Check sheet for the drawn part. Datum: minimum x, y, z corner. Units: mm. Coordinates: 2 decimals unless noted, no trailing zeros. Write each loop counter-clockwise with the first axis right and the second up, starting at its lowest first coordinate (ties: lowest second). Pieces come first, ordered by that corner, then holes. Notation, with made-up numbers: (85.25, 17) -> (131.25, 17) arc R34 cw to (131.25, 51) -> close; hole circle Ø6 at (25, 87.25). An arc over 180 degrees is marked (long way). Answer in a Markdown table with one row per item. Add a question column.
1. Cross-section at B-B on z = 2.1. Record the cut outline in (x, y), and give its area (3 significant figures).
2. Cross-section at D-D on z = 0.35. Record the cut outline in (x, y), and give its area (3 significant figures).
3. Cross-section at A-A on y = 3.75. Record the cut outline in (x, z).
4. Depth check by flat-ended pin: P1, Ø1, axis at x = 3, z = 1, coming from the -Y side; P2, Ø1, axis at x = 2, z = 1, coming from the +Y side. Enter the tip coordinate at first touch or a pass-through.
5. Cross-section at C-C on z = 1.65. Record the cut outline in (x, y).
6. Scan lines: L1, parallel to Y at x = 3.75, z = 1.15; L2, parallel to Z at x = 2.25, y = 4.5; L3, parallel to X at y = 5.25, z = 0.25. Record each from-to range of solid material in increasing order. Write a range as from..to.
7. Mould release check, pull along Y, two halves, no side actions. Record for the marked faces 1, 2 and 3: pulls with the +Y half, pulls with the -Y half, needs draft (parallel to the pull), parting line crosses it, or undercut.
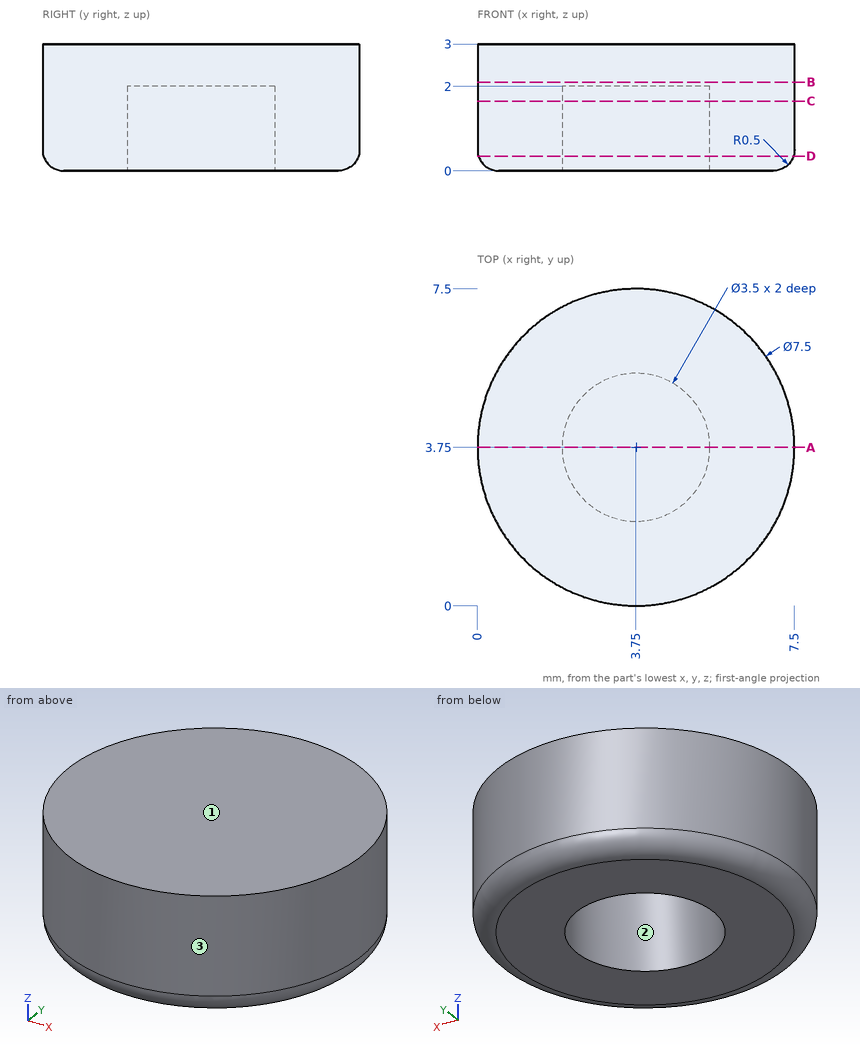
Results found:
| question | item | result |
|---|---|---|
| 1 | outline | circle Ø7.5 at (3.75, 3.75) |
| 1 | area | 44.2 mm^2 |
| 2 | outline | circle Ø7.45 at (3.75, 3.75); hole circle Ø3.5 at (3.75, 3.75) |
| 2 | area | 34.0 mm^2 |
| 3 | outline | (0, 0.5) arc R0.5 ccw to (0.5, 0) -> (2, 0) -> (2, 2) -> (5.5, 2) -> (5.5, 0) -> (7, 0) arc R0.5 ccw to (7.5, 0.5) -> (7.5, 3) -> (0, 3) -> close |
| 4 | P1 | stops at y = 0.01 |
| 4 | P2 | stops at y = 7.29 |
| 5 | outline | circle Ø7.5 at (3.75, 3.75); hole circle Ø3.5 at (3.75, 3.75) |
| 6 | L1 | y = 0..2, 5.5..7.5 |
| 6 | L2 | z = 2..3 |
| 6 | L3 | x = 0.39..2.85, 4.65..7.11 |
| 7 | face 1 | needs draft |
| 7 | face 2 | undercut |
| 7 | face 3 | parting line crosses it |
